Design review of the part built by this model. Coordinates are the model's own, in mm. Face numbers are marked on the shaded views. A direction names the side the tool comes from. Give positions to 0.01 mm unless a question says otherwise; leave off trailing zeros. Write each loop counter-clockwise with the first axis right and the second up, starting at its lowest first coordinate (ties: lowest second). Pieces come first, ordered by that corner, then holes. Notation, with made-up numbers: M -29.75,33.25 L -23.75,33.25 A28 ccw -23.75,62.25 Z; hole C 69.25,-34.75 d8. An arc over 180 degrees is marked long. Answer in a Markdown table with one row per item.
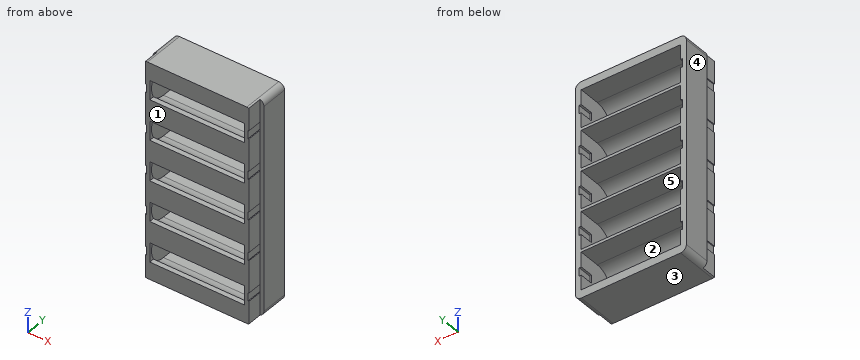
```python
from build123d import *

# Parameters (mm, degrees)
SKETCH_241_W                = 95.8
SKETCH_241_H                = 36.6
EXTRUDE_326_DEPTH           = 36.6
CUT_EXTRUDE_START           = -5
SKETCH_380_R                = 16.3
CUT_EXTRUDE_539_DEPTH       = 85.8
SKETCH_588_W                = 85.8
SKETCH_588_H                = 32.6
CUT_EXTRUDE_850_DEPTH       = 18.3
CUT_EXTRUDE_1245_DEPTH      = 109.888750567
CUT_EXTRUDE_1245_DEPTH_BACK = 109.888750567
SKETCH_902_W                = 0.75
SKETCH_902_H                = 7.1
SKETCH_A_W                  = 7.1
SKETCH_A_H                  = 11.6
CUT_EXTRUDE_A_DEPTH         = 1
SKETCH_B_W                  = 7.1
SKETCH_B_H                  = 11.6
CUT_EXTRUDE_B_DEPTH         = 1
SKETCH_1779_W               = 81.8
SKETCH_1779_H               = 16.6
CUT_EXTRUDE_2059_DEPTH      = 109.888750567
SKETCH_2105_W               = 3.25
SKETCH_2105_H               = 13.1
CUT_EXTRUDE_2527_DEPTH      = 13
PATTERN_LINEAR_2584_COUNT   = 5
PATTERN_LINEAR_2584_PITCH   = 35
SKETCH_2694_W               = 95.8
SKETCH_2694_H               = 36.6
EXTRUDE_2884_DEPTH          = 5
SKETCH_2964_W               = 95.8
SKETCH_2964_H               = 36.6
EXTRUDE_3079_DEPTH          = 5
FILLET_1_R                  = 5
FILLET_2_R                  = 5
FILLET_3_R                  = 5
FILLET_4_R                  = 5
SKETCH_3561_W               = 186.6
SKETCH_3561_H               = 13
CUT_EXTRUDE_3822_DEPTH      = 3.25
SKETCH_4173_W               = 186.6
SKETCH_4173_H               = 13
CUT_EXTRUDE_4352_DEPTH      = 3.25


with BuildPart() as part:
    # Sketch 241 → Extrude 326 (new body)
    with BuildSketch(Plane(origin=(0, 0, 0), x_dir=(1, 0, 0), z_dir=(0, 1, 0))):
        with Locations((-47.9, 18.3)):
            Rectangle(SKETCH_241_W, SKETCH_241_H)
    extrude(amount=EXTRUDE_326_DEPTH)

    # Sketch 380 → Cut-Extrude 539 (cut)
    with BuildSketch(Plane(origin=(0, 0, 0), x_dir=(0, 0, -1), z_dir=(1, 0, 0)).offset(CUT_EXTRUDE_START)):
        with Locations((18.3, 18.3)):
            Circle(SKETCH_380_R)
    extrude(amount=-CUT_EXTRUDE_539_DEPTH, mode=Mode.SUBTRACT)

    # Sketch 588 → Cut-Extrude 850 (cut)
    with BuildSketch(Plane(origin=(0, 36.6, 0), x_dir=(1, 0, 0), z_dir=(0, 1, 0))):
        with Locations((-47.9, 18.3)):
            Rectangle(SKETCH_588_W, SKETCH_588_H)
    extrude(amount=-CUT_EXTRUDE_850_DEPTH, mode=Mode.SUBTRACT)

    # Sketch 902 → Cut-Extrude 1245 (cut, two sides: drawn at the far end of the back side and taken through both)
    with BuildSketch(Plane(origin=(0, 36.6, 0), x_dir=(1, 0, 0), z_dir=(0, 1, 0)).offset(-CUT_EXTRUDE_1245_DEPTH_BACK)):
        with Locations((-92.175, 18.3)):
            Rectangle(SKETCH_902_W, SKETCH_902_H)
        with Locations((-3.625, 18.3)):
            Rectangle(SKETCH_902_W, SKETCH_902_H)
    extrude(amount=CUT_EXTRUDE_1245_DEPTH + CUT_EXTRUDE_1245_DEPTH_BACK, mode=Mode.SUBTRACT)

    # 触点开窗面A → 触点开窗A (cut)
    with BuildSketch(Plane(origin=(-90.8, 0, 0), x_dir=(0, 0, -1), z_dir=(1, 0, 0))):
        with Locations((18.3, 30.8)):
            Rectangle(SKETCH_A_W, SKETCH_A_H)
    extrude(amount=-CUT_EXTRUDE_A_DEPTH, mode=Mode.SUBTRACT)

    # 触点开窗面B → 触点开窗B (cut)
    with BuildSketch(Plane.ZY.offset(5)):
        with Locations((-18.3, 30.8)):
            Rectangle(SKETCH_B_W, SKETCH_B_H)
    extrude(amount=-CUT_EXTRUDE_B_DEPTH, mode=Mode.SUBTRACT)

    # Sketch 1779 → Cut-Extrude 2059 (cut, through all)
    with BuildSketch(Plane.XZ):
        with Locations((-47.9, -18.3)):
            Rectangle(SKETCH_1779_W, SKETCH_1779_H)
    extrude(amount=-CUT_EXTRUDE_2059_DEPTH, mode=Mode.SUBTRACT)

    # Sketch 2105 → Cut-Extrude 2527 (cut)
    with BuildSketch(Plane.XZ):
        with Locations((-94.175, -18.3)):
            Rectangle(SKETCH_2105_W, SKETCH_2105_H)
        with Locations((-1.625, -18.3)):
            Rectangle(SKETCH_2105_W, SKETCH_2105_H)
    extrude(amount=-CUT_EXTRUDE_2527_DEPTH, mode=Mode.SUBTRACT)


with BuildPart() as pattern_linear_2584_1:
    # Pattern Linear 2584: pattern copy
    add(part.part.moved(Location(Vector(0, 0, -1) * (1 * PATTERN_LINEAR_2584_PITCH))))


with BuildPart() as pattern_linear_2584_2:
    # Pattern Linear 2584: pattern copy
    add(part.part.moved(Location(Vector(0, 0, -1) * (2 * PATTERN_LINEAR_2584_PITCH))))


with BuildPart() as pattern_linear_2584_3:
    # Pattern Linear 2584: pattern copy
    add(part.part.moved(Location(Vector(0, 0, -1) * (3 * PATTERN_LINEAR_2584_PITCH))))


with BuildPart() as pattern_linear_2584_4:
    # Pattern Linear 2584: pattern copy
    add(part.part.moved(Location(Vector(0, 0, -1) * (4 * PATTERN_LINEAR_2584_PITCH))))

    # Sketch 2694 → Extrude 2884 (add)
    with BuildSketch(Plane(origin=(0, 0, -176.6), x_dir=(-1, 0, 0), z_dir=(0, 0, -1))):
        with Locations((47.9, 18.3)):
            Rectangle(SKETCH_2694_W, SKETCH_2694_H)
    extrude(amount=EXTRUDE_2884_DEPTH)

    # 圆角3
    fillet_3_edges = [pattern_linear_2584_4.edges().sort_by_distance(p)[0] for p in [
        (-95.8, 18.3, -181.6),
    ]]
    fillet(fillet_3_edges, radius=FILLET_3_R)

    # 圆角4
    fillet_4_edges = [pattern_linear_2584_4.edges().sort_by_distance(p)[0] for p in [
        (0, 18.3, -181.6),
    ]]
    fillet(fillet_4_edges, radius=FILLET_4_R)


with BuildPart() as part_1:
    add(part.part)

    # Sketch 2964 → Extrude 3079 (add)
    with BuildSketch(Plane.XY):
        with Locations((-47.9, 18.3)):
            Rectangle(SKETCH_2964_W, SKETCH_2964_H)
    extrude(amount=EXTRUDE_3079_DEPTH)

    # 圆角1
    fillet_1_edges = [part_1.edges().sort_by_distance(p)[0] for p in [
        (-95.8, 18.3, 5),
    ]]
    fillet(fillet_1_edges, radius=FILLET_1_R)

    # 圆角2
    fillet_2_edges = [part_1.edges().sort_by_distance(p)[0] for p in [
        (0, 18.3, 5),
    ]]
    fillet(fillet_2_edges, radius=FILLET_2_R)


with BuildPart() as cut_extrude_3822_tool:
    # Sketch 3561 → Cut-Extrude 3822 (new body)
    with BuildSketch(Plane.ZY.offset(95.8)):
        with Locations((-88.3, 6.5)):
            Rectangle(SKETCH_3561_W, SKETCH_3561_H)
    extrude(amount=-CUT_EXTRUDE_3822_DEPTH)


with BuildPart() as part_2:
    add(part_1.part)

    # Cut-Extrude 3822: cut by cut_extrude_3822_tool
    add(cut_extrude_3822_tool.part, mode=Mode.SUBTRACT)


with BuildPart() as pattern_linear_2584_1_1:
    add(pattern_linear_2584_1.part)

    # Cut-Extrude 3822: cut by cut_extrude_3822_tool
    add(cut_extrude_3822_tool.part, mode=Mode.SUBTRACT)


with BuildPart() as pattern_linear_2584_2_1:
    add(pattern_linear_2584_2.part)

    # Cut-Extrude 3822: cut by cut_extrude_3822_tool
    add(cut_extrude_3822_tool.part, mode=Mode.SUBTRACT)


with BuildPart() as pattern_linear_2584_3_1:
    add(pattern_linear_2584_3.part)

    # Cut-Extrude 3822: cut by cut_extrude_3822_tool
    add(cut_extrude_3822_tool.part, mode=Mode.SUBTRACT)


with BuildPart() as pattern_linear_2584_4_1:
    add(pattern_linear_2584_4.part)

    # Cut-Extrude 3822: cut by cut_extrude_3822_tool
    add(cut_extrude_3822_tool.part, mode=Mode.SUBTRACT)


with BuildPart() as cut_extrude_4352_tool:
    # Sketch 4173 → Cut-Extrude 4352 (new body)
    with BuildSketch(Plane(origin=(0, 0, 0), x_dir=(0, 0, -1), z_dir=(1, 0, 0))):
        with Locations((88.3, 6.5)):
            Rectangle(SKETCH_4173_W, SKETCH_4173_H)
    extrude(amount=-CUT_EXTRUDE_4352_DEPTH)


with BuildPart() as part_3:
    add(part_2.part)

    # Cut-Extrude 4352: cut by cut_extrude_4352_tool
    add(cut_extrude_4352_tool.part, mode=Mode.SUBTRACT)


with BuildPart() as pattern_linear_2584_1_2:
    add(pattern_linear_2584_1_1.part)

    # Cut-Extrude 4352: cut by cut_extrude_4352_tool
    add(cut_extrude_4352_tool.part, mode=Mode.SUBTRACT)


with BuildPart() as pattern_linear_2584_2_2:
    add(pattern_linear_2584_2_1.part)

    # Cut-Extrude 4352: cut by cut_extrude_4352_tool
    add(cut_extrude_4352_tool.part, mode=Mode.SUBTRACT)


with BuildPart() as pattern_linear_2584_3_2:
    add(pattern_linear_2584_3_1.part)

    # Cut-Extrude 4352: cut by cut_extrude_4352_tool
    add(cut_extrude_4352_tool.part, mode=Mode.SUBTRACT)


with BuildPart() as pattern_linear_2584_4_2:
    add(pattern_linear_2584_4_1.part)

    # Cut-Extrude 4352: cut by cut_extrude_4352_tool
    add(cut_extrude_4352_tool.part, mode=Mode.SUBTRACT)


with BuildPart() as pattern_linear_2584_1_3:
    add(pattern_linear_2584_1_2.part)

    # Combine 5S: union Pattern Linear 2584_2, Pattern Linear 2584_3, Pattern Linear 2584_4, part
    add(pattern_linear_2584_2_2.part)
    add(pattern_linear_2584_3_2.part)
    add(pattern_linear_2584_4_2.part)
    add(part_3.part)


solid = pattern_linear_2584_1_3.part
```
1) Add section B-B (y = 34). Count the separate pieces of the cut face and the enclosed holes in it, and give its area (3 significant figures).
Geometry says:
| item | result |
|---|---|
| separate pieces | 1 |
| enclosed holes | 5 |
| area | 3,750 mm^2 |
2) The part is to be moulded in two halves that separate along Z. For the marked faces 1, 2 and 3, say which applies: released by +Z, released by -Z, zero draft, split by the parting line, or undercut.
Geometry says:
| item | result |
|---|---|
| face 1 | zero draft |
| face 2 | undercut |
| face 3 | released by -Z |
3) Add section A-A (z = -88.3). Write out the cut boundary in (x, y).
Geometry says:
| item | result |
|---|---|
| outline | M -95.8,13 L -92.55,13 L -92.55,36.6 L -95.8,36.6 Z; M -91.8,0 L -88.8,0 L -88.8,2 L -90.8,2 L -90.8,25 L -91.8,25 Z; M -7,0 L -4,0 L -4,25 L -5,25 L -5,2 L -7,2 Z; M -3.25,13 L 0,13 L 0,36.6 L -3.25,36.6 Z |
4) Add section D-D (z = -111.5). Write out the cut boundary in (x, y) (3 decimals).
Geometry says:
| item | result |
|---|---|
| outline | M -95.8,13 L -92.55,13 L -92.55,0 L -3.25,0 L -3.25,13 L 0,13 L 0,36.6 L -5,36.6 L -5,7.055 L -90.8,7.055 L -90.8,36.6 L -95.8,36.6 Z |
5) To check wall thickness, follow probe 1 along Z at (x, y) = (-64.5, 24.5); probe 2 along X at (y, z) = (35, -8.5); probe 3 along X at (y, z) = (4.5, -88). State the ranges of each line that lie inside material, in increasing order. Write a range as [from, to].
Geometry says:
| item | result |
|---|---|
| probe 1 | [-181.6, -174.6], [-142, -139.6], [-107, -104.6], [-72, -69.6], [-37, -34.6], [-2, 5] |
| probe 2 | [-95.8, -90.8], [-5, 0] |
| probe 3 | [-91.8, -90.8], [-5, -4] |
6) For the marked faces 4 and 5, list the 3-axis set-ups (+Z, -Z, +X, -X, +Y, -Y) from which the entire face can be reached by the end or side of a thin tool; tool diameter is ignored.
Geometry says:
| item | result |
|---|---|
| face 4 | +Z, -Z, -X, +Y, -Y |
| face 5 | +Y |
7) Insertion check: P1, Ø0.5, axis at x = -4.5, y = 18, coming from the -Z side; P2, Ø3.5, axis at y = 10.5, z = -53, coming from the -X side; P3, Ø3, axis at x = -69.5, z = -41.5, coming from the -Y side; P4, Ø1, axis at x = -62, z = -145, coming from the +Y side. Each pin has a flat end and moves straight along its axis. Give the tip position at first contact, or say it passes through.
Geometry says:
| item | result |
|---|---|
| P1 | z = -181.59 |
| P2 | x = -91.8 |
| P3 | y = 0 |
| P4 | y = 9.63 |
